from build123d import *

# Parameters (mm, degrees)
IZIM1_W                      = 30
IZIM1_H                      = 130
TABAN_FLAN_1_DEPTH           = 1.5
RADYUS1_R                    = 10
KENAR_FLAN_1_STRIP_W         = 12
KENAR_FLAN_1_STRIP_H         = 1.5
KENAR_FLAN_1_STRIP_CUT_DEPTH = 130
KENAR_FLAN_1_DEPTH           = 130
KENAR_START                  = -53.051470588
KENAR_EKME1_DEPTH            = 130
KENAR_EKME1_2_DEPTH          = 130
RADYUS2_R                    = 5


# Read off the part's stored shape, not the designer's step: Kenar Çekme1
# Sheet-metal steps are written as plain solids
with BuildPart() as part:
    # Çizim1 → Taban-Flanş1 (new body)
    with BuildSketch(Plane.XY):
        with Locations((-32.781930006, 11.948529412)):
            Rectangle(IZIM1_W, IZIM1_H)
    extrude(amount=-TABAN_FLAN_1_DEPTH)

    # Radyus1
    radyus1_edges = [part.edges().sort_by_distance(p)[0] for p in [
        (-17.781930006, 76.948529412, -0.75),
        (-17.781930006, -53.051470588, -0.75),
    ]]
    fillet(radyus1_edges, radius=RADYUS1_R)

    # Kenar-Flanş1 strip (across the edge) → Kenar-Flanş1 strip cut (cut)
    with BuildSketch(Plane(origin=(-47.781930006, 76.948529412, 0), x_dir=(1, 0, 0), z_dir=(0, -1, 0))):
        with Locations((-1.5, -0.75)):
            Rectangle(KENAR_FLAN_1_STRIP_W, KENAR_FLAN_1_STRIP_H)
    extrude(amount=KENAR_FLAN_1_STRIP_CUT_DEPTH, mode=Mode.SUBTRACT)

    # Kenar-Flanş1 section (across the edge) → Kenar-Flanş1 (add)
    with BuildSketch(Plane(origin=(-47.781930006, 76.948529412, 0), x_dir=(1, 0, 0), z_dir=(0, -1, 0))):
        with BuildLine():
            Line((0, 3), (0, 18))
            Line((0, 18), (1.5, 18))
            Line((1.5, 18), (1.5, 3))
            ThreePointArc((1.5, 3), (2.378679656, 0.878679656), (4.5, 0))
            Line((4.5, 0), (4.5, -1.5))
            ThreePointArc((4.5, -1.5), (1.318019485, -0.181980515), (0, 3))
        make_face()
    extrude(amount=KENAR_FLAN_1_DEPTH)

    # Kenar Çekme1 outline → Kenar Çekme1 (cut)
    with BuildSketch(Plane(origin=(0, 0, 0), x_dir=(1, 0, 0), z_dir=(0, 1, 0)).offset(KENAR_START)):
        with BuildLine():
            ThreePointArc((-46.281930006, -15.25), (-46.686722126, -16.686140662), (-47.781930006, -17.699489743))
            Line((-47.781930006, -17.699489743), (-47.781930006, -18))
            Line((-47.781930006, -18), (-46.281930006, -18))
            Line((-46.281930006, -18), (-46.281930006, -15.25))
        make_face()
    extrude(amount=KENAR_EKME1_DEPTH, mode=Mode.SUBTRACT)

    # Kenar _ekme1 2 outline → Kenar _ekme1 2 (add)
    with BuildSketch(Plane(origin=(0, 0, 0), x_dir=(1, 0, 0), z_dir=(0, 1, 0)).offset(KENAR_START)):
        with BuildLine():
            Line((-50.281930006, -5), (-51.781930006, -5))
            Line((-51.781930006, -5), (-51.781930006, -15.25))
            ThreePointArc((-51.781930006, -15.25), (-50.468070668, -17.59520788), (-47.781930006, -17.699489743))
            Line((-47.781930006, -17.699489743), (-47.781930006, -15.25))
            ThreePointArc((-47.781930006, -15.25), (-49.031930006, -16.5), (-50.281930006, -15.25))
            Line((-50.281930006, -15.25), (-50.281930006, -5))
        make_face()
    extrude(amount=KENAR_EKME1_2_DEPTH)

    # Radyus2
    radyus2_edges = [part.edges().sort_by_distance(p)[0] for p in [
        (-51.031930006, 76.948529412, 5),
        (-51.031930006, -53.051470588, 5),
    ]]
    fillet(radyus2_edges, radius=RADYUS2_R)


solid = part.part
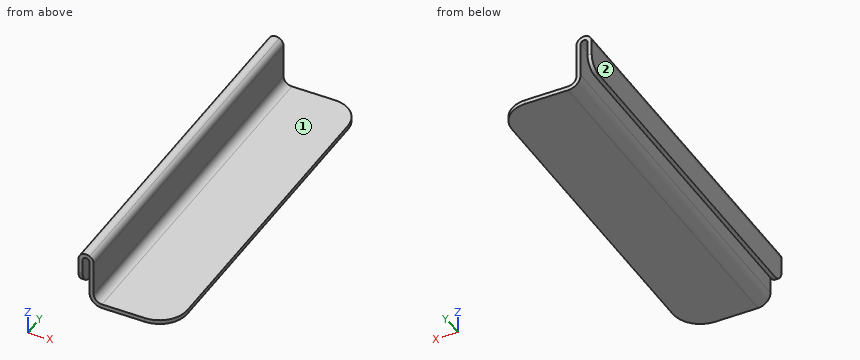
Model file for the job. Use its own axes, mm. Face numbers are marked on the shaded views. A direction names the side the tool comes from. Give positions to 0.01 mm unless a question says otherwise; leave off trailing zeros. Write each loop counter-clockwise with the first axis right and the second up, starting at its lowest first coordinate (ties: lowest second). Pieces come first, ordered by that corner, then holes. Notation, with made-up numbers: M 50.5,15.5 L 88.5,15.5 A20 cw 88.5,25.5 Z; hole C 54,39 d2. An arc over 180 degrees is marked long. One line per item, written item: value. Start each with the question number.
Q1. 3-axis set-ups, long thin cutter, end or side, ignore diameter. For the marked faces 1 and 2: which of +Z, -Z, +X, -X, +Y, -Y reach the whole face in a straight line?
Q2. Saw through at B-B, the plane z = 8.5. Write the cut outline in (x, y), plus the area to 3 significant figures.
Q3. Probe probe 1 along X at (y, z) = (18, 7.5); probe 2 along Z at (x, y) = (-30, 7); probe 3 along X at (y, z) = (-21, 4.5). List the from-to ranges inside material, lowest first. Write a range as [from, to].
Q4. Saw through at D-D, the plane x = -25. Write the cut outline in (y, z), plus the area to 3 significant figures.
Q5. Saw through at C-C, the plane x = -36.5. Write the cut outline in (y, z), plus the area to 3 significant figures.
Q6. Saw through at A-A, the plane y = -2. Write the cut outline in (x, z).
Q7. Drop flat-ended pins along their axis: pin 1 Ø3 at (y, z) = (-24.5, 7) entering from +X; pin 2 Ø2 at (y, z) = (-21, 2.5) entering from -X; pin 3 Ø10 at (x, z) = (-36, 8.5) entering from +Y; pin 4 Ø1.5 at (x, y) = (-24, -28) entering from +Z. Give the stop position or say it passes through.
Output values:
1. face 1: +Z, +X, +Y, -Y
1. face 2: +Z, -Z, -X, +Y, -Y
2. outline: M -51.78,-52.82 L -50.28,-52.82 L -50.28,76.72 L -51.78,76.72 Z; M -47.78,-53.05 L -46.28,-53.05 L -46.28,76.95 L -47.78,76.95 Z
2. area: 389 mm²
3. probe 1: x = [-51.78, -50.28], [-47.78, -46.28]
3. probe 2: z = [-1.5, 0]
3. probe 3: x = [-47.78, -46.28]
4. outline: M -52.66,-1.5 L 76.55,-1.5 L 76.55,0 L -52.66,0 Z
4. area: 194 mm²
5. outline: M -53.05,-1.5 L 76.95,-1.5 L 76.95,0 L -53.05,0 Z
5. area: 195 mm²
6. outline: M -51.78,5 L -50.28,5 L -50.28,15.25 A1.25 cw -47.78,15.25 L -47.78,3 A4.5 ccw -43.28,-1.5 L -17.78,-1.5 L -17.78,0 L -43.28,0 A3 cw -46.28,3 L -46.28,15.25 A2.75 ccw -51.78,15.25 Z
7. pin 1: stops at x = -46.28
7. pin 2: stops at x = -47.78
7. pin 3: passes through
7. pin 4: stops at z = 0
